Verification items for the finished model (mm, model axes). A direction names the side the tool comes from. Round coordinates to 2 decimals unless told otherwise and drop trailing zeros. Write each loop counter-clockwise with the first axis right and the second up, starting at its lowest first coordinate (ties: lowest second). Pieces come first, ordered by that corner, then holes.
Autodesk Inventor part; units mm, degrees
ref_plane "YZ Plane" through (0, 0, 0) normal (1, 0, 0) x (0, 1, 0)
ref_plane "XZ Plane" through (0, 0, 0) normal (0, 1, 0) x (-1, 0, 0)
ref_plane "XY Plane" through (0, 0, 0) normal (0, 0, 1) x (1, 0, 0)
sketch "Sketch1" plane through (0, 0, 0) normal (0, 0, 1) x (1, 0, 0)
  circle A0 centre (25.625, 0) radius 1.5125
  line L0 (12.5, 21.35) -> (0, 21.35)
  line L1 (0, -20.65) -> (0, 28.35) construction
  line L2 (-39.7989, 0) -> (39.7989, 0) construction
  line L3 (27.3095, -2.1737) -> (12.5, -13.65)
  line L4 (12.5, -13.65) -> (0, -13.65)
  arc A1 (27.3095, -2.1737) -> (27.2023, 2.2527) centre (25.625, 0) ccw
  circle A2 centre (-25.625, 0) radius 1.5125
  line L5 (-12.5, 21.35) -> (0, 21.35)
  line L6 (-27.3095, -2.1737) -> (-12.5, -13.65)
  line L7 (-12.5, -13.65) -> (0, -13.65)
  arc A3 (-27.2023, 2.2527) -> (-27.3095, -2.1737) centre (-25.625, 0) ccw
  line L8 (27.2023, 2.2527) -> (18.625, 8.2586)
  line L9 (18.625, 8.2586) -> (12.5, 21.35)
  line L10 (-27.2023, 2.2527) -> (-18.625, 8.2586)
  line L11 (-18.625, 8.2586) -> (-12.5, 21.35)
  point P0 (0, 0)
  dimension "d0" = 51.25
  dimension "d1" = 3.025
  dimension "d2" = 2.75
  dimension "d84" = 21.35
  dimension "d85" = 13.65
  dimension "d86" = 25
  dimension "d87" = 25
  dimension "d88" = 35
  dimension "d89" = 7
extrude "Extrusion1" add sketch "Sketch1" along normal blind 5
sketch "Sketch4" plane through (0, 0, 5) normal (0, 0, 1) x (1, 0, 0)
  line L0 (-39.725, 0) -> (39.725, 0) construction
  line L1 (0, -20.65) -> (0, 28.35) construction
  point P0 (0, 0)
  point P1 (9.5, -10.5)
  point P2 (8, 18.5)
  point P3 (-6, 18.5)
  point P4 (-9.5, -10.5)
  dimension "d90" = 10.5
  dimension "d91" = 9.5
  dimension "d92" = 18.5
  dimension "d93" = 18.5
  dimension "d94" = 8
  dimension "d95" = 6
hole "Hole2" at (9.5, -10.5, 5) at (8, 18.5, 5) at (-6, 18.5, 5) at (-9.5, -10.5, 5) direction (0, 0, -1) diameter 2.2 end through all counterbore diameter 4 counterbore depth 2
fillet "Fillet5" radius 2 6 edges at (-18.625, 8.2586, 2.5) (18.625, 8.2586, 2.5) (12.5, -13.65, 2.5) (-12.5, -13.65, 2.5) (12.5, 21.35, 2.5) (-12.5, 21.35, 2.5)
chamfer "Chamfer4" distance 0.3 angle 45 44 edges at (0, 21.35, 5) (-12.3012, 21.0375, 5) (-15.7188, 14.4701, 5) (-18.6787, 8.3037, 5) (-23.1326, 5.1023, 5) (-28.3742, 0.0665, 5) (12.3012, 21.0375, 5) (15.7188, 14.4701, 5) (18.6787, 8.3037, 5) (23.1326, 5.1023, 5) (28.3742, 0.0665, 5) (0, 21.35, 0) (12.3012, 21.0375, 0) (15.7188, 14.4701, 0) (18.6787, 8.3037, 0) (23.1326, 5.1023, 0) (28.3742, 0.0665, 0) (-12.3012, 21.0375, 0) (-15.7188, 14.4701, 0) (-18.6787, 8.3037, 0) (-23.1326, 5.1023, 0) (-28.3742, 0.0665, 0) (-20.1752, -7.7023, 5) (-12.4632, -13.5423, 5) (0, -13.65, 5) (12.4632, -13.5423, 5) (20.1752, -7.7023, 5) (-20.1752, -7.7023, 0) (-12.4632, -13.5423, 0) (0, -13.65, 0) (12.4632, -13.5423, 0) (20.1752, -7.7023, 0) (-27.1375, 0, 0) (-9.5, -9.4, 0) (9.5, -9.4, 0) (-6, 19.6, 0) (8, 19.6, 0) (24.1125, 0, 0) (-27.1375, 0, 5) (24.1125, 0, 5) (-9.5, -8.5, 5) (9.5, -8.5, 5) (-6, 20.5, 5) (8, 20.5, 5)
equation "\"d0\" = dist_hinge_points"
equation "\"d1\" = bore_clearance"
equation "\"d104\" = champfer"
equation "\"finger_width\" = 25"
equation "\"finger_thickness\" = 8"
equation "\"finger_part_A_length\" = 42.8625"
equation "\"finger_part_B_length\" = 28.575"
equation "\"finger_link_width\" = 3.5"
equation "\"finger_link_clearence\" = 0.075"
equation "\"tol\" = 0.5 * finger_link_clearence"
equation "\"link_tol\" = 0.254"
equation "\"bore_press\" = 2.925"
equation "\"bore_clearance\" = 3.025"
equation "\"bar_diameter\" = 6.5"
equation "\"bar_thickness\" = 4"
equation "\"bar_width\" = 7"
equation "\"hinge_dist_sym_plane\" = 4"
equation "\"hinge_thickness\" = 3"
equation "\"hinge_act_length_c\" = 7.62"
equation "\"hinge_act_length_bc\" = 16.66875"
equation "\"hinge_act_length_ab\" = 11.049"
equation "\"hinge_act_length_a\" = 21.43125"
equation "\"hinge_guid_length_c\" = 9.525"
equation "\"hinge_guid_length_bc\" = 9.525"
equation "\"hinge_guid_length_ab\" = 17.145"
equation "\"hinge_guid_length_a\" = 17.145"
equation "\"bar_length_bc\" = finger_part_B_length"
equation "\"bar_act_length_ab\" = 40.48125"
equation "\"bar_guid_length_ab\" = 43.275"
equation "\"champfer\" = 0.3"
equation "\"fillet\" = 0.4"
equation "\"hinge_point\" = 15"
equation "\"dist_finger_BC\" = 56.5"
equation "\"gear_diameter\" = 14"
properties part number "tilt-guide"
Q1. Sectioned sample at B-B (z = 1.1). Give the number of separate pieces and of enclosed holes in the cut face, plus the area to 3 significant figures.
Recorded:
separate pieces: 1
enclosed holes: 6
area: 1,360 mm2
Q2. Material ranges on line 1 along X through (y, z) = (-10.5, 1.4); line 2 along X through (y, z) = (-10.5, 3.4); line 3 along Y through (x, z) = (-6, 3.7), recorded low to high.
Recorded:
line 1: x = -16.56 to -10.6, -8.4 to 8.4, 10.6 to 16.56
line 2: x = -16.56 to -11.5, -7.5 to 7.5, 11.5 to 16.56
line 3: y = -13.65 to 16.5, 20.5 to 21.35
Q3. Sectioned sample at D-D (y = 11). Enter the section's corners in (x, z).
Recorded:
outline: (-17.34, 0.3) - (-17.01, 0) - (17.01, 0) - (17.34, 0.3) - (17.34, 4.7) - (17.01, 5) - (-17.01, 5) - (-17.34, 4.7) - close
Q4. Tool access check on faces 1 (the cylindrical face through (8, 19.6, 1.6)), 2 (the cylindrical face through (6.648, 19.974, 3.838)). Record the directions out of +Z, -Z, +X, -X, +Y, -Y that give a thin tool (end or side, any length) a straight path to the whole face; none if there is none.
Recorded:
face 1: +Z, -Z
face 2: +Z
Q5. Depth check by flat-ended pin: P1, Ø3, axis at x = 8, y = 18.5, coming from the -Z side; P2, Ø2.5, axis at x = 25.625, y = 0, coming from the +Z side; P3, Ø3, axis at x = -9, y = -11, coming from the +Z side; P4, Ø2, axis at y = 9.5, z = 2, coming from the +X side. Enter the tip coordinate at first touch or a pass-through.
Recorded:
P1: stops at z = 0
P2: passes through
P3: stops at z = 4.91
P4: stops at x = 18.53
Q6. Release check for a two-part mould opening along Y. For faces 3 (the flat face through (15.62, 14.33, 4.85)), 4 (the cylindrical face through (-27.136, -0.067, 2.469)), 5 (the cylindrical face through (-28.375, 0.031, 2.469)) record: released by +Y, released by -Y, zero draft, split by the parting line, or undercut.
Recorded:
face 3: released by +Y
face 4: undercut
face 5: split by the parting line
Q7. Sectioned sample at A-A (x = -9.5). Enter the section's corners in (y, z), plus the area to 3 significant figures.
Recorded:
outline: (-13.65, 0.3) - (-13.35, 0) - (-11.9, 0) - (-11.6, 0.3) - (-11.6, 3) - (-12.5, 3) - (-12.5, 4.7) - (-12.8, 5) - (-13.35, 5) - (-13.65, 4.7) - close; (-9.4, 0.3) - (-9.1, 0) - (21.05, 0) - (21.35, 0.3) - (21.35, 4.7) - (21.05, 5) - (-8.2, 5) - (-8.5, 4.7) - (-8.5, 3) - (-9.4, 3) - close
area: 160 mm2
